from build123d import *

# Parameters (mm, degrees)
SKETCH1_R           = 2.5
SKETCH1_R_2         = 1
SKETCH1_W           = 6.5
SKETCH1_H           = 3.5
BOSS_EXTRUDE1_DEPTH = 3


with BuildPart() as part:
    # Sketch1 → Boss-Extrude1 (new body)
    with BuildSketch(Plane(origin=(0, 0, 0), x_dir=(1, 0, 0), z_dir=(0, 1, 0))):
        with BuildLine():
            Line((-32.25, 45), (32.25, 45))
            ThreePointArc((32.25, 45), (32.729781285, 45.011516135), (33.208457525, 45.046038016))
            Line((33.208457525, 45.046038016), (65.158413836, 48.122468899))
            ThreePointArc((65.158413836, 48.122468899), (67.665203844, 48.696022601), (69.942838419, 49.88989895))
            ThreePointArc((69.942838419, 49.88989895), (81.731024928, 44.283166046), (70.857119505, 37.061325846))
            ThreePointArc((70.857119505, 37.061325846), (68.189665999, 37.969274319), (65.374821319, 38.097055623))
            Line((65.374821319, 38.097055623), (38.671218724, 35.525791146))
            ThreePointArc((38.671218724, 35.525791146), (34.907627779, 33.194274373), (34.470507151, 28.788651508))
            ThreePointArc((34.470507151, 28.788651508), (35.099285854, 27.2130238), (35.790444846, 25.663745072))
            ThreePointArc((35.790444846, 25.663745072), (35.738430228, 24.716138108), (34.918224383, 24.238721256))
            ThreePointArc((34.918224383, 24.238721256), (33.203553641, 23.478673593), (32.5, 21.740059064))
            Line((32.5, 21.740059064), (32.5, -21.740059064))
            ThreePointArc((32.5, -21.740059064), (33.203553641, -23.478673593), (34.918224383, -24.238721256))
            ThreePointArc((34.918224383, -24.238721256), (35.738430228, -24.716138108), (35.790444846, -25.663745072))
            ThreePointArc((35.790444846, -25.663745072), (35.099285854, -27.2130238), (34.470507151, -28.788651508))
            ThreePointArc((34.470507151, -28.788651508), (34.907627779, -33.194274373), (38.671218724, -35.525791146))
            Line((38.671218724, -35.525791146), (65.374821319, -38.097055623))
            ThreePointArc((65.374821319, -38.097055623), (68.189665999, -37.969274319), (70.857119505, -37.061325846))
            ThreePointArc((70.857119505, -37.061325846), (81.731024928, -44.283166046), (69.942838419, -49.88989895))
            ThreePointArc((69.942838419, -49.88989895), (67.665203844, -48.696022601), (65.158413836, -48.122468899))
            Line((65.158413836, -48.122468899), (33.208457525, -45.046038016))
            ThreePointArc((33.208457525, -45.046038016), (32.729781285, -45.011516135), (32.25, -45))
            Line((32.25, -45), (-32.25, -45))
            ThreePointArc((-32.25, -45), (-32.729781285, -45.011516135), (-33.208457525, -45.046038016))
            Line((-33.208457525, -45.046038016), (-65.158413836, -48.122468899))
            ThreePointArc((-65.158413836, -48.122468899), (-67.665203844, -48.696022601), (-69.942838419, -49.88989895))
            ThreePointArc((-69.942838419, -49.88989895), (-81.731024928, -44.283166046), (-70.857119505, -37.061325846))
            ThreePointArc((-70.857119505, -37.061325846), (-68.189665999, -37.969274319), (-65.374821319, -38.097055623))
            Line((-65.374821319, -38.097055623), (-38.671218724, -35.525791146))
            ThreePointArc((-38.671218724, -35.525791146), (-34.907627779, -33.194274373), (-34.470507151, -28.788651508))
            ThreePointArc((-34.470507151, -28.788651508), (-35.099285854, -27.2130238), (-35.790444846, -25.663745072))
            ThreePointArc((-35.790444846, -25.663745072), (-35.738430228, -24.716138108), (-34.918224383, -24.238721256))
            ThreePointArc((-34.918224383, -24.238721256), (-33.203553641, -23.478673593), (-32.5, -21.740059064))
            Line((-32.5, -21.740059064), (-32.5, 21.740059064))
            ThreePointArc((-32.5, 21.740059064), (-33.203553641, 23.478673593), (-34.918224383, 24.238721256))
            ThreePointArc((-34.918224383, 24.238721256), (-35.738430228, 24.716138108), (-35.790444846, 25.663745072))
            ThreePointArc((-35.790444846, 25.663745072), (-35.099285854, 27.2130238), (-34.470507151, 28.788651508))
            ThreePointArc((-34.470507151, 28.788651508), (-34.907627779, 33.194274373), (-38.671218724, 35.525791146))
            Line((-38.671218724, 35.525791146), (-65.374821319, 38.097055623))
            ThreePointArc((-65.374821319, 38.097055623), (-68.189665999, 37.969274319), (-70.857119505, 37.061325846))
            ThreePointArc((-70.857119505, 37.061325846), (-81.731024928, 44.283166046), (-69.942838419, 49.88989895))
            ThreePointArc((-69.942838419, 49.88989895), (-67.665203844, 48.696022601), (-65.158413836, 48.122468899))
            Line((-65.158413836, 48.122468899), (-33.208457525, 45.046038016))
            ThreePointArc((-33.208457525, 45.046038016), (-32.729781285, 45.011516135), (-32.25, 45))
        make_face()
        with Locations(Location((74.25, 43.75, 0), (0, 0, 270))):
            Circle(SKETCH1_R, mode=Mode.SUBTRACT)
        with Locations(Location((70.777689375, 46.612351991, 0), (0, 0, 270))):
            Circle(SKETCH1_R_2, mode=Mode.SUBTRACT)
        with Locations(Location((77.112351991, 47.222310625, 0), (0, 0, 270))):
            Circle(SKETCH1_R_2, mode=Mode.SUBTRACT)
        with Locations(Location((77.722310625, 40.887648009, 0), (0, 0, 270))):
            Circle(SKETCH1_R_2, mode=Mode.SUBTRACT)
        with Locations(Location((71.387648009, 40.277689375, 0), (0, 0, 270))):
            Circle(SKETCH1_R_2, mode=Mode.SUBTRACT)
        with Locations(Location((-71.387648009, 40.277689375, 0), (0, 0, 90))):
            Circle(SKETCH1_R_2, mode=Mode.SUBTRACT)
        with Locations(Location((-77.722310625, 40.887648009, 0), (0, 0, 90))):
            Circle(SKETCH1_R_2, mode=Mode.SUBTRACT)
        with Locations(Location((-77.112351991, 47.222310625, 0), (0, 0, 90))):
            Circle(SKETCH1_R_2, mode=Mode.SUBTRACT)
        with Locations(Location((-70.777689375, 46.612351991, 0), (0, 0, 90))):
            Circle(SKETCH1_R_2, mode=Mode.SUBTRACT)
        with Locations(Location((-74.25, 43.75, 0), (0, 0, 90))):
            Circle(SKETCH1_R, mode=Mode.SUBTRACT)
        with Locations(Location((-74.25, -43.75, 0), (0, 0, 270))):
            Circle(SKETCH1_R, mode=Mode.SUBTRACT)
        with Locations(Location((-70.777689375, -46.612351991, 0), (0, 0, 270))):
            Circle(SKETCH1_R_2, mode=Mode.SUBTRACT)
        with Locations(Location((-77.112351991, -47.222310625, 0), (0, 0, 270))):
            Circle(SKETCH1_R_2, mode=Mode.SUBTRACT)
        with Locations(Location((-77.722310625, -40.887648009, 0), (0, 0, 270))):
            Circle(SKETCH1_R_2, mode=Mode.SUBTRACT)
        with Locations(Location((-71.387648009, -40.277689375, 0), (0, 0, 270))):
            Circle(SKETCH1_R_2, mode=Mode.SUBTRACT)
        with Locations(Location((71.387648009, -40.277689375, 0), (0, 0, 90))):
            Circle(SKETCH1_R_2, mode=Mode.SUBTRACT)
        with Locations(Location((77.722310625, -40.887648009, 0), (0, 0, 90))):
            Circle(SKETCH1_R_2, mode=Mode.SUBTRACT)
        with Locations(Location((77.112351991, -47.222310625, 0), (0, 0, 90))):
            Circle(SKETCH1_R_2, mode=Mode.SUBTRACT)
        with Locations(Location((70.777689375, -46.612351991, 0), (0, 0, 90))):
            Circle(SKETCH1_R_2, mode=Mode.SUBTRACT)
        with Locations(Location((74.25, -43.75, 0), (0, 0, 90))):
            Circle(SKETCH1_R, mode=Mode.SUBTRACT)
        with BuildLine():
            Line((-17.6, 39), (17.6, 39))
            ThreePointArc((17.6, 39), (18.559559999, 38.28150419), (18.14024032, 37.158489218))
            Line((18.14024032, 37.158489218), (0.54024032, 25.859490032))
            ThreePointArc((0.54024032, 25.859490032), (0, 25.701000814), (-0.54024032, 25.859490032))
            Line((-0.54024032, 25.859490032), (-18.14024032, 37.158489218))
            ThreePointArc((-18.14024032, 37.158489218), (-18.559559999, 38.28150419), (-17.6, 39))
        make_face(mode=Mode.SUBTRACT)
        with BuildLine():
            Line((4, 1.5), (25.5, 1.5))
            ThreePointArc((25.5, 1.5), (26.207106781, 1.792893219), (26.5, 2.5))
            Line((26.5, 2.5), (26.5, 18))
            ThreePointArc((26.5, 18), (26.207106781, 18.707106781), (25.5, 19))
            Line((25.5, 19), (4, 19))
            ThreePointArc((4, 19), (3.292893219, 18.707106781), (3, 18))
            Line((3, 18), (3, 2.5))
            ThreePointArc((3, 2.5), (3.292893219, 1.792893219), (4, 1.5))
        make_face(mode=Mode.SUBTRACT)
        with Locations((17.75, 23.75)):
            Rectangle(SKETCH1_W, SKETCH1_H, mode=Mode.SUBTRACT)
        with Locations((-17.75, 23.75)):
            Rectangle(SKETCH1_W, SKETCH1_H, mode=Mode.SUBTRACT)
        with BuildLine():
            Line((-26.5, 2.5), (-26.5, 18))
            ThreePointArc((-26.5, 18), (-26.207106781, 18.707106781), (-25.5, 19))
            Line((-25.5, 19), (-4, 19))
            ThreePointArc((-4, 19), (-3.292893219, 18.707106781), (-3, 18))
            Line((-3, 18), (-3, 2.5))
            ThreePointArc((-3, 2.5), (-3.292893219, 1.792893219), (-4, 1.5))
            Line((-4, 1.5), (-25.5, 1.5))
            ThreePointArc((-25.5, 1.5), (-26.207106781, 1.792893219), (-26.5, 2.5))
        make_face(mode=Mode.SUBTRACT)
        with BuildLine():
            Line((-4, -1.5), (-25.5, -1.5))
            ThreePointArc((-25.5, -1.5), (-26.207106781, -1.792893219), (-26.5, -2.5))
            Line((-26.5, -2.5), (-26.5, -18))
            ThreePointArc((-26.5, -18), (-26.207106781, -18.707106781), (-25.5, -19))
            Line((-25.5, -19), (-4, -19))
            ThreePointArc((-4, -19), (-3.292893219, -18.707106781), (-3, -18))
            Line((-3, -18), (-3, -2.5))
            ThreePointArc((-3, -2.5), (-3.292893219, -1.792893219), (-4, -1.5))
        make_face(mode=Mode.SUBTRACT)
        with Locations((-17.75, -23.75)):
            Rectangle(SKETCH1_W, SKETCH1_H, mode=Mode.SUBTRACT)
        with BuildLine():
            Line((-18.14024032, -37.158489218), (-0.54024032, -25.859490032))
            ThreePointArc((-0.54024032, -25.859490032), (0, -25.701000814), (0.54024032, -25.859490032))
            Line((0.54024032, -25.859490032), (18.14024032, -37.158489218))
            ThreePointArc((18.14024032, -37.158489218), (18.559559999, -38.28150419), (17.6, -39))
            Line((17.6, -39), (-17.6, -39))
            ThreePointArc((-17.6, -39), (-18.559559999, -38.28150419), (-18.14024032, -37.158489218))
        make_face(mode=Mode.SUBTRACT)
        with Locations((17.75, -23.75)):
            Rectangle(SKETCH1_W, SKETCH1_H, mode=Mode.SUBTRACT)
        with BuildLine():
            Line((26.5, -2.5), (26.5, -18))
            ThreePointArc((26.5, -18), (26.207106781, -18.707106781), (25.5, -19))
            Line((25.5, -19), (4, -19))
            ThreePointArc((4, -19), (3.292893219, -18.707106781), (3, -18))
            Line((3, -18), (3, -2.5))
            ThreePointArc((3, -2.5), (3.292893219, -1.792893219), (4, -1.5))
            Line((4, -1.5), (25.5, -1.5))
            ThreePointArc((25.5, -1.5), (26.207106781, -1.792893219), (26.5, -2.5))
        make_face(mode=Mode.SUBTRACT)
    extrude(amount=BOSS_EXTRUDE1_DEPTH)


solid = part.part
The model under review builds one solid part; all positions refer to its coordinate system, in mm. A direction names the side the tool comes from. Round coordinates to 2 decimals unless told otherwise and drop trailing zeros. Loops run counter-clockwise (first coordinate to the right, second up) from the corner with the lowest first, then second, coordinate; pieces in that order, holes last. Notation, with made-up numbers: (-36, 35) - (-15, 35) arc R19 ccw to (-15, 60) - close; hole circle Ø11 at (-0.75, 31). An arc over 180 degrees is marked (long way). Use CSV: the item, a comma, the result in double quotes.
(1) Machinability: for faces 4 (the flat face through (-15, 1, -19)), 5 (the flat face through (0, 1, 45)), 6 (the flat face through (32.5, 1, 0)), which of the approach directions +Z, -Z, +X, -X, +Y, -Y give a long, thin tool a straight path to every point of the face, cutting with its end or side? Answer none if there is none.
Working result:
face 4,"+Y, -Y"
face 5,"+Z, +Y, -Y"
face 6,"+X, +Y, -Y"
(2) For line 1 (X direction, y = 2, z = -17.5); line 2 (Z direction, x = -74.5, y = 1.9); line 3 (Z direction, x = -1.5, y = 1.55), list the stretches that pass through material, from the lowest coordinate up.
Working result:
line 1,"x = -32.5 to -26.5, -3 to 3, 26.5 to 32.5"
line 2,"z = -51.25 to -46.24, -41.26 to -36.25, 36.25 to 41.26, 46.24 to 51.25"
line 3,"z = -45 to -39, -26.48 to 26.48, 39 to 45"
(3) The part is to be moulded in two halves that separate along Z. For faces 1 (the cylindrical face through (76.47, 1.48, 42.6)), 2 (the cylindrical face through (-67.631, 1.479, 48.684)), 3 (the flat face through (-49.407, 1.479, -46.606)), say which applies: pulls with the +Z half, pulls with the -Z half, needs draft (parallel to the pull), parting line crosses it, or undercut.
Working result:
face 1,"undercut"
face 2,"pulls with the +Z half"
face 3,"pulls with the -Z half"
(4) Take a section at A-A, the plane z = 9.5. Give the boundary of the cut face in (x, y).
Working result:
outline,"(-32.5, 0) - (-26.5, 0) - (-26.5, 3) - (-32.5, 3) - close; (-3, 0) - (3, 0) - (3, 3) - (-3, 3) - close; (26.5, 0) - (32.5, 0) - (32.5, 3) - (26.5, 3) - close"
(5) Take a section at D-D, the plane x = 44. Give the boundary of the cut face in (y, z).
Working result:
outline,"(0, -46.09) - (3, -46.09) - (3, -36.04) - (0, -36.04) - close; (0, 36.04) - (3, 36.04) - (3, 46.09) - (0, 46.09) - close"
(6) Take a section at C-C, the plane x = 23. Give the boundary of the cut face in (y, z), plus the area to 3 significant figures.
Working result:
outline,"(0, -45) - (3, -45) - (3, -19) - (0, -19) - close; (0, -1.5) - (3, -1.5) - (3, 1.5) - (0, 1.5) - close; (0, 19) - (3, 19) - (3, 45) - (0, 45) - close"
area,"165 mm^2"
(7) Take a section at B-B, the plane x = -74.25. Give the boundary of the cut face in (y, z), plus the area to 3 significant figures.
Working result:
outline,"(0, -51.25) - (3, -51.25) - (3, -46.25) - (0, -46.25) - close; (0, -41.25) - (3, -41.25) - (3, -36.25) - (0, -36.25) - close; (0, 36.25) - (3, 36.25) - (3, 41.25) - (0, 41.25) - close; (0, 46.25) - (3, 46.25) - (3, 51.25) - (0, 51.25) - close"
area,"60.0 mm^2"
(8) Clearance check with flat-ended pins moving along their axes: P1, Ø1.5, axis at y = 1.5, z = 5.5, coming from the -X side; P2, Ø0.9, axis at y = 2, z = 24, coming from the +X side; P3, Ø1.6, axis at x = 70.78, z = 46.61, coming from the -Y side; P4, Ø1.5, axis at y = 1, z = -10, coming from the +X side. State where each tip first meets the part, or that it passes through.
Working result:
P1,"stops at x = -32.5"
P2,"stops at x = 35.5"
P3,"passes through"
P4,"stops at x = 32.5"
